Design review of the part built by this model. Coordinates are the model's own, in mm. Face numbers are marked on the shaded views. Coordinates: 2 decimals unless noted, no trailing zeros. Loops run counter-clockwise (first coordinate to the right, second up) from the corner with the lowest first, then second, coordinate; pieces in that order, holes last. Notation, with made-up numbers: (3, 50.25) -> (23, 50.25) arc R20 ccw to (23, 71.25) -> close; hole circle Ø4 at (22, 16.5). An arc over 180 degrees is marked (long way). Use CSV: the item, a comma, the result in double quotes.
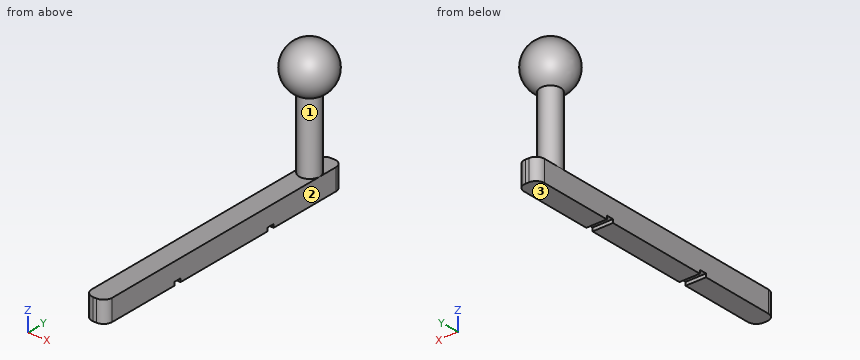
```python
from build123d import *

# Parameters (mm, degrees)
F1_DEPTH = 7.5
F2_W     = 7.2
F2_H     = 2.6
F3_DEPTH = 1.2
F4_R     = 3.6
F5_DEPTH = 25


with BuildPart() as f1:
    # F0 (on Top) → F1 (new body)
    with BuildSketch(Plane.XY):
        with BuildLine():
            ThreePointArc((3.6, 46.75), (2.72132, 48.87132), (0.6, 49.75))
            Line((0.6, 49.75), (-0.6, 49.75))
            ThreePointArc((-0.6, 49.75), (-2.72132, 48.87132), (-3.6, 46.75))
            Line((-3.6, 46.75), (-3.6, -46.75))
            ThreePointArc((-3.6, -46.75), (-2.72132, -48.87132), (-0.6, -49.75))
            Line((-0.6, -49.75), (0.6, -49.75))
            ThreePointArc((0.6, -49.75), (2.72132, -48.87132), (3.6, -46.75))
            Line((3.6, -46.75), (3.6, 46.75))
        make_face()
    extrude(amount=F1_DEPTH)

    # F2 (on face) → F3 (cut)
    with BuildSketch(Plane(origin=(0, 0, 0), x_dir=(1, 0, 0), z_dir=(0, 0, -1))):
        with Locations((0, 19.45)):
            Rectangle(F2_W, F2_H)
        with Locations((0, -19.45)):
            Rectangle(F2_W, F2_H)
    extrude(amount=-F3_DEPTH, mode=Mode.SUBTRACT)

    # F4 (on face) → F5 (join)
    with BuildSketch(Plane.XY.offset(7.5)):
        with Locations((0, 40)):
            Circle(F4_R)
    extrude(amount=F5_DEPTH)

    # F7 (on offset) → F8 (revolve)
    with BuildSketch(Plane.XZ.offset(-40)):
        with BuildLine():
            Line((0, 31.55), (0, 48.45))
            ThreePointArc((0, 48.45), (-8.45, 40), (0, 31.55))
        make_face()
    revolve(axis=Axis((0, 40, 40), (0, 0, 1)))


solid = f1.part
```
Item 1: Add section A-A (x = 1.5). Give the boundary of the cut face in (y, z), then the cut area to 3 significant figures.
Checked values:
outline,"(-49.61, 0) -> (-20.75, 0) -> (-20.75, 1.2) -> (-18.15, 1.2) -> (-18.15, 0) -> (18.15, 0) -> (18.15, 1.2) -> (20.75, 1.2) -> (20.75, 0) -> (49.61, 0) -> (49.61, 7.5) -> (43.27, 7.5) -> (43.27, 32.36) arc R8.32 ccw (long way) to (36.73, 32.36) -> (36.73, 7.5) -> (-49.61, 7.5) -> close"
area,"1,110 mm^2"
Item 2: Clearance check with flat-ended pins moving along their axes: pin 1 (0.8 mm diameter, centred on x = 1, y = 19, fed in from -Z); pin 2 (5 mm diameter, centred on x = 1.5, z = 17.5, fed in from +Y); pin 3 (1.5 mm diameter, centred on x = -1.5, z = 29, fed in from +Y). State where each tip first meets the part, or that it passes through.
Checked values:
pin 1,"z = 1.2"
pin 2,"y = 43.6"
pin 3,"y = 43.52"
Item 3: To check wall thickness, follow line 1 along Z through (x, y) = (-1.5, -27.5); line 2 along X through (y, z) = (44.5, 3.5); line 3 along Z through (x, y) = (1, 35.5). State the ranges of each line that lie inside material, in increasing order.
Checked values:
line 1,"0 to 7.5"
line 2,"-3.6 to 3.6"
line 3,"0 to 7.5, 32.92 to 47.08"
Item 4: Add section D-D (x = -2.5). Give the boundary of the cut face in (y, z).
Checked values:
outline,"(-49.07, 0) -> (-20.75, 0) -> (-20.75, 1.2) -> (-18.15, 1.2) -> (-18.15, 0) -> (18.15, 0) -> (18.15, 1.2) -> (20.75, 1.2) -> (20.75, 0) -> (49.07, 0) -> (49.07, 7.5) -> (42.59, 7.5) -> (42.59, 32.36) arc R8.07 ccw (long way) to (37.41, 32.36) -> (37.41, 7.5) -> (-49.07, 7.5) -> close"
Item 5: Add section B-B (z = 10). Give the boundary of the cut face in (x, y), then the cut area to 3 significant figures.
Checked values:
outline,"circle Ø7.2 at (0, 40)"
area,"40.7 mm^2"
Item 6: Add section C-C (y = -24). Give the boundary of the cut face in (x, z).
Checked values:
outline,"(-3.6, 0) -> (3.6, 0) -> (3.6, 7.5) -> (-3.6, 7.5) -> close"
Item 7: Draft analysis for pull direction Z (two halves, no side actions). For the marked faces 1, 2 and 3, state which applies: pulls with the +Z half, pulls with the -Z half, needs draft (parallel to the pull), parting line crosses it, or undercut.
Checked values:
face 1,"undercut"
face 2,"needs draft"
face 3,"pulls with the -Z half"
